```python
from build123d import *

# Parameters (mm, degrees)
SKETCH1_R           = 12
BOSS_EXTRUDE1_DEPTH = 6
CUT_EXTRUDE1_REACH  = 91.29
SKETCH2_R           = 1.5
CUT_EXTRUDE2_REACH  = 91.29
SKETCH3_R           = 1.5
FILLET1_R           = 1.5


with BuildPart() as part:
    # Sketch1 → Boss-Extrude1 (new body)
    with BuildSketch(Plane(origin=(0, 0, 0), x_dir=(0, 0, -1), z_dir=(1, 0, 0))):
        with BuildLine():
            Line((68.0694084, 0), (0, 0))
            Line((0, 0), (0, -10))
            Line((0, -10), (10, -10))
            Line((10, -10), (10, -33.439310345))
            ThreePointArc((10, -33.439310345), (34.0347042, -57.474014545), (58.0694084, -33.439310345))
            Line((58.0694084, -33.439310345), (58.0694084, -10))
            Line((58.0694084, -10), (68.0694084, -10))
            Line((68.0694084, -10), (68.0694084, 0))
        make_face()
        with Locations((34.0347042, -33.439310345)):
            Circle(SKETCH1_R, mode=Mode.SUBTRACT)
    extrude(amount=BOSS_EXTRUDE1_DEPTH)

    # Sketch2 → Cut-Extrude1 (cut, up to next)
    with BuildSketch(Plane(origin=(0, 0, 0), x_dir=(1, 0, 0), z_dir=(0, 1, 0)), mode=Mode.PRIVATE) as cut_extrude1_sk1:
        with Locations(Location((3, 63.0694084, 0), (0, 0, 270))):
            Circle(SKETCH2_R)
    cut_extrude1_tool1 = extrude(cut_extrude1_sk1.sketch, amount=-CUT_EXTRUDE1_REACH, mode=Mode.PRIVATE) & part.part
    # Sketch2 → Cut-Extrude1 (cut, up to next)
    with BuildSketch(Plane(origin=(0, 0, 0), x_dir=(1, 0, 0), z_dir=(0, 1, 0)), mode=Mode.PRIVATE) as cut_extrude1_sk2:
        with BuildLine():
            ThreePointArc((3.771743633, 6.286239389), (1.713760611, 5.771743633), (2.228256367, 3.713760611))
            Line((2.228256367, 3.713760611), (3.771743633, 6.286239389))
        make_face()
    cut_extrude1_tool2 = extrude(cut_extrude1_sk2.sketch, amount=-CUT_EXTRUDE1_REACH, mode=Mode.PRIVATE) & part.part
    # Sketch2 → Cut-Extrude1 (cut, up to next)
    with BuildSketch(Plane(origin=(0, 0, 0), x_dir=(1, 0, 0), z_dir=(0, 1, 0)), mode=Mode.PRIVATE) as cut_extrude1_sk3:
        with BuildLine():
            Line((3.771743633, 6.286239389), (2.228256367, 3.713760611))
            ThreePointArc((2.228256367, 3.713760611), (3.739048222, 3.69470014), (4.5, 5))
            ThreePointArc((4.5, 5), (4.30529986, 5.739048222), (3.771743633, 6.286239389))
        make_face()
    cut_extrude1_tool3 = extrude(cut_extrude1_sk3.sketch, amount=-CUT_EXTRUDE1_REACH, mode=Mode.PRIVATE) & part.part
    # Sketch2 → Cut-Extrude1 (cut, up to next)
    with BuildSketch(Plane(origin=(0, 0, 0), x_dir=(1, 0, 0), z_dir=(0, 1, 0)), mode=Mode.PRIVATE) as cut_extrude1_sk4:
        with BuildLine():
            ThreePointArc((3.771743633, 6.286239389), (1.713760611, 5.771743633), (2.228256367, 3.713760611))
            Line((2.228256367, 3.713760611), (3.771743633, 6.286239389))
        make_face()
    cut_extrude1_tool4 = extrude(cut_extrude1_sk4.sketch, amount=-CUT_EXTRUDE1_REACH, mode=Mode.PRIVATE) & part.part
    # Sketch2 → Cut-Extrude1 (cut, up to next)
    with BuildSketch(Plane(origin=(0, 0, 0), x_dir=(1, 0, 0), z_dir=(0, 1, 0)), mode=Mode.PRIVATE) as cut_extrude1_sk5:
        with BuildLine():
            Line((3.771743633, 6.286239389), (2.228256367, 3.713760611))
            ThreePointArc((2.228256367, 3.713760611), (3.739048222, 3.69470014), (4.5, 5))
            ThreePointArc((4.5, 5), (4.30529986, 5.739048222), (3.771743633, 6.286239389))
        make_face()
    cut_extrude1_tool5 = extrude(cut_extrude1_sk5.sketch, amount=-CUT_EXTRUDE1_REACH, mode=Mode.PRIVATE) & part.part
    add(cut_extrude1_tool1.solids().sort_by_distance((3, 0, -63.069408))[0], mode=Mode.SUBTRACT)
    add(cut_extrude1_tool2.solids().sort_by_distance((2.454103, 0, -5.327538))[0], mode=Mode.SUBTRACT)
    add(cut_extrude1_tool3.solids().sort_by_distance((3.545897, 0, -4.672462))[0], mode=Mode.SUBTRACT)
    add(cut_extrude1_tool4.solids().sort_by_distance((2.454103, 0, -5.327538))[0], mode=Mode.SUBTRACT)
    add(cut_extrude1_tool5.solids().sort_by_distance((3.545897, 0, -4.672462))[0], mode=Mode.SUBTRACT)

    # Sketch3 → Cut-Extrude2 (cut, up to next)
    with BuildSketch(Plane(origin=(0, 0, 0), x_dir=(0, 0, -1), z_dir=(1, 0, 0)), mode=Mode.PRIVATE) as cut_extrude2_sk1:
        with Locations((42.0347042, -47.295716805)):
            Circle(SKETCH3_R)
    cut_extrude2_tool1 = extrude(cut_extrude2_sk1.sketch, amount=CUT_EXTRUDE2_REACH, mode=Mode.PRIVATE) & part.part
    # Sketch3 → Cut-Extrude2 (cut, up to next)
    with BuildSketch(Plane(origin=(0, 0, 0), x_dir=(0, 0, -1), z_dir=(1, 0, 0)), mode=Mode.PRIVATE) as cut_extrude2_sk2:
        with Locations((50.0347042, -33.439310345)):
            Circle(SKETCH3_R)
    cut_extrude2_tool2 = extrude(cut_extrude2_sk2.sketch, amount=CUT_EXTRUDE2_REACH, mode=Mode.PRIVATE) & part.part
    # Sketch3 → Cut-Extrude2 (cut, up to next)
    with BuildSketch(Plane(origin=(0, 0, 0), x_dir=(0, 0, -1), z_dir=(1, 0, 0)), mode=Mode.PRIVATE) as cut_extrude2_sk3:
        with Locations((26.0347042, -19.582903884)):
            Circle(SKETCH3_R)
    cut_extrude2_tool3 = extrude(cut_extrude2_sk3.sketch, amount=CUT_EXTRUDE2_REACH, mode=Mode.PRIVATE) & part.part
    # Sketch3 → Cut-Extrude2 (cut, up to next)
    with BuildSketch(Plane(origin=(0, 0, 0), x_dir=(0, 0, -1), z_dir=(1, 0, 0)), mode=Mode.PRIVATE) as cut_extrude2_sk4:
        with Locations((18.0347042, -33.439310345)):
            Circle(SKETCH3_R)
    cut_extrude2_tool4 = extrude(cut_extrude2_sk4.sketch, amount=CUT_EXTRUDE2_REACH, mode=Mode.PRIVATE) & part.part
    # Sketch3 → Cut-Extrude2 (cut, up to next)
    with BuildSketch(Plane(origin=(0, 0, 0), x_dir=(0, 0, -1), z_dir=(1, 0, 0)), mode=Mode.PRIVATE) as cut_extrude2_sk5:
        with Locations((42.0347042, -19.582903884)):
            Circle(SKETCH3_R)
    cut_extrude2_tool5 = extrude(cut_extrude2_sk5.sketch, amount=CUT_EXTRUDE2_REACH, mode=Mode.PRIVATE) & part.part
    # Sketch3 → Cut-Extrude2 (cut, up to next)
    with BuildSketch(Plane(origin=(0, 0, 0), x_dir=(0, 0, -1), z_dir=(1, 0, 0)), mode=Mode.PRIVATE) as cut_extrude2_sk6:
        with Locations((26.0347042, -47.295716805)):
            Circle(SKETCH3_R)
    cut_extrude2_tool6 = extrude(cut_extrude2_sk6.sketch, amount=CUT_EXTRUDE2_REACH, mode=Mode.PRIVATE) & part.part
    add(cut_extrude2_tool1.solids().sort_by_distance((0, -47.295717, -42.034704))[0], mode=Mode.SUBTRACT)
    add(cut_extrude2_tool2.solids().sort_by_distance((0, -33.43931, -50.034704))[0], mode=Mode.SUBTRACT)
    add(cut_extrude2_tool3.solids().sort_by_distance((0, -19.582904, -26.034704))[0], mode=Mode.SUBTRACT)
    add(cut_extrude2_tool4.solids().sort_by_distance((0, -33.43931, -18.034704))[0], mode=Mode.SUBTRACT)
    add(cut_extrude2_tool5.solids().sort_by_distance((0, -19.582904, -42.034704))[0], mode=Mode.SUBTRACT)
    add(cut_extrude2_tool6.solids().sort_by_distance((0, -47.295717, -26.034704))[0], mode=Mode.SUBTRACT)

    # Fillet1
    fillet1_edges = [part.edges().sort_by_distance(p)[0] for p in [
        (3, 0, -68.0694084),
        (3, 0, 0),
        (3, -10, -68.0694084),
        (3, -10, 0),
        (3, -10, -58.0694084),
        (3, -10, -10),
    ]]
    fillet(fillet1_edges, radius=FILLET1_R)


solid = part.part
```
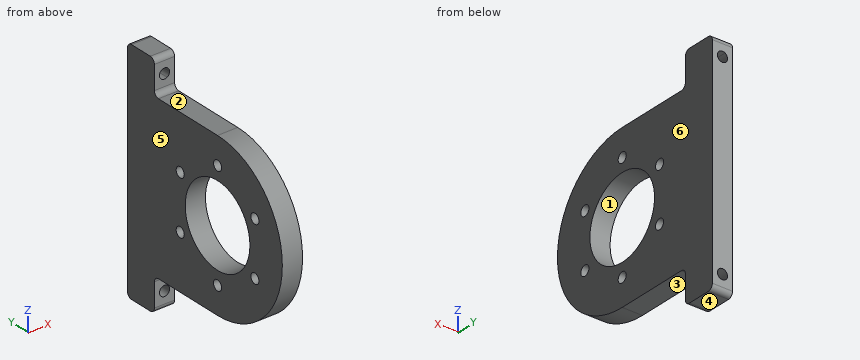
Verification items for the finished model (mm, model axes). Face numbers are marked on the shaded views. A direction names the side the tool comes from. Coordinates: 2 decimals unless noted, no trailing zeros. Write each loop counter-clockwise with the first axis right and the second up, starting at its lowest first coordinate (ties: lowest second). Pieces come first, ordered by that corner, then holes. Notation, with made-up numbers: (-23.5, 80.25) - (2.5, 80.25) arc R14 cw to (2.5, 106.25) - close; hole circle Ø11 at (-33.5, 61.5). An arc over 180 degrees is marked (long way). Write item = value, one per line.
Q1. Access from +Z, -Z, +X, -X, +Y, -Y to the whole of each face (thin tool, end or side, straight path). Record for the marked faces 1, 2 and 3.
Answer:
face_1 = +X, -X
face_2 = +Z, +X, -X, -Y
face_3 = -Z, +X, -X, -Y
Q2. Cross-section at A-A (x = 3). Give the number of separate pieces and of enclosed holes in the cut face, plus the area to 3 significant figures.
Answer:
separate_pieces = 3
enclosed_holes = 7
area = 2,160 mm²
Q3. Cross-section at B-B (y = -30). Enter the section's corners in (x, z), plus the area to 3 significant figures.
Answer:
outline = (0, -58.07) - (6, -58.07) - (6, -45.53) - (0, -45.53) - close; (0, -22.54) - (6, -22.54) - (6, -10) - (0, -10) - close
area = 150 mm²
Q4. Cross-section at D-D (y = -16). Enter the section's corners in (x, z).
Answer:
outline = (0, -58.07) - (6, -58.07) - (6, -10) - (0, -10) - close
Q5. Go/stop test with flat-tipped pins: pin 1 Ø1.8 at (y, z) = (-47.3, -42.03) entering from -X; pin 2 Ø3.5 at (x, z) = (3, -63.07) entering from -Y; pin 3 Ø1.8 at (x, y) = (4.5, -18) entering from -Z; pin 4 Ø2 at (x, z) = (3.5, -12) entering from -Y. Record where each tip stops, or that it passes through.
Answer:
pin_1 = through
pin_2 = -10
pin_3 = -58.07
pin_4 = -45.07
Q6. Material ranges on L1, parallel to Z at x = 3.2, y = -33; L2, parallel to Y at x = 1.9, z = -8; L3, parallel to Z at x = 1.3, y = -13.5, recorded low to high. Write a range as from..to.
Answer:
L1 = -58.07..-51.47, -48.6..-46.03, -22.04..-19.47, -16.6..-10
L2 = -10..0
L3 = -58.07..-10
Q7. Cross-section at C-C (z = -33). Enter the section's corners in (x, y), plus the area to 3 significant figures.
Answer:
outline = (0, -57.45) - (6, -57.45) - (6, -45.39) - (0, -45.39) - close; (0, -21.48) - (6, -21.48) - (6, 0) - (0, 0) - close
area = 201 mm²
Q8. Mould release check, pull along X, two halves, no side actions. Record for the marked faces 4, 5 and 6: released by +X, released by -X, zero draft, split by the parting line, or undercut.
Answer:
face_4 = zero draft
face_5 = released by -X
face_6 = released by +X
